Can you work these out from the model? Positions are in its coordinate system, mm. A direction names the side the tool comes from. Give positions to 0.01 mm unless a question says otherwise; leave off trailing zeros. Order: outer loops, then holes, each group sorted by start corner. A loop starts at its lowest first (then second) coordinate and runs counter-clockwise, first axis right, second up.
Item 1: I want a section at A-A, the plane y = 21.5. Write out the boundary of the cut face in (x, z), then the cut area to 3 significant figures.
Item 2: I want a section at B-B, the plane z = 3.75. Write out the boundary of the cut face in (x, y).
Item 3: If we mould it in two halves opening along Y, with no side actions, what happens to faces 1 (the flat face through (33, 0, 5.08)), 2 (the cylindrical face through (53.944, 47.249, 3.792)), 3 (the cylindrical face through (18.98, -15.5, 6.86)), 4 (the flat face through (48, 31, 2.54))? For each: +Y half, -Y half, draft (parallel to the pull), parting line (faces both ways), or undercut.
Item 4: I'm going to push flat-ended pins straight in: pin 1 Ø5.5 at (x, y) = (33, 2.5) entering from -Z; pin 2 Ø1.5 at (x, z) = (43.5, 1) entering from +Y; pin 3 Ø2 at (x, z) = (28.5, 3) entering from +Y; pin 4 Ø12 at (x, y) = (8, 10) entering from +Z. Where does each tip first touch, or does it pass through?
Item 5: Which directions (+Z, -Z, +X, -X, +Y, -Y) give clear straight access to the entire face, cutting with the end or side of a thin tool? Please do faces 5 (the cylindrical face through (9.436, 23.933, 0.764)), 6 (the cylindrical face through (23.98, 61.47, 3.79)), 7 (the flat face through (0, 24, 4)), 8 (the flat face through (49.32, 34.14, 6.33)).
Item 6: If I drill on line 1 along X through (y, z) = (23.5, 5.25); line 2 along Y through (x, z) = (43.5, 3); line 3 along Y through (x, z) = (17, 7.25), over which ranges is the centre line in solid material (lowest first)?
```python
from build123d import *

# Parameters (mm, degrees)
BOSS_EXTRUDE1_DEPTH     = 7.62
FILLET1_R               = 2.54
SKETCH4_W               = 10.16
SKETCH4_H               = 2.54
BOSS_EXTRUDE2_DEPTH     = 40.698655059
CUT_EXTRUDE1_DEPTH      = 92.035139481
CUT_EXTRUDE1_DEPTH_BACK = 92.035139481
SKETCH7_R               = 1.27
CUT_EXTRUDE2_DEPTH      = 92.212140759


with BuildPart() as part:
    # Sketch2 → Boss-Extrude1 (new body)
    with BuildSketch(Plane.XY):
        with BuildLine():
            Line((557.368573337, 914.592873905), (556.734884655, 913.276848696))
            Line((556.734884655, 913.276848696), (547.580835245, 917.684680294))
            Line((547.580835245, 917.684680294), (548.214523926, 919.000705503))
            ThreePointArc((548.214523926, 919.000705503), (548.458818056, 919.731374997), (548.513066645, 920.499889552))
            ThreePointArc((548.513066645, 920.499889552), (547.585939227, 924.379743345), (545.358485968, 927.689015574))
            ThreePointArc((545.358485968, 927.689015574), (538.788952643, 934.173311823), (531.958551893, 940.382216038))
            ThreePointArc((531.958551893, 940.382216038), (526.80512603, 942.791823737), (521.15870091, 942.097640216))
            ThreePointArc((521.15870091, 942.097640216), (515.269866914, 937.194322522), (513.062812413, 929.85608018))
            Line((513.062812413, 929.85608018), (513.062812413, 881.310664403))
            ThreePointArc((513.062812413, 881.310664403), (514.84238247, 877.01697918), (519.13757646, 875.241053792))
            Line((519.13757646, 875.241053792), (524.686345009, 875.245763006))
            ThreePointArc((524.686345009, 875.245763006), (526.769666342, 875.847420281), (528.214212618, 877.464672677))
            Line((528.214212618, 877.464672677), (529.924061844, 881.015635083))
            Line((529.924061844, 881.015635083), (539.078111254, 876.607803485))
            Line((539.078111254, 876.607803485), (537.368262028, 873.056841079))
            ThreePointArc((537.368262028, 873.056841079), (532.178962974, 867.247123196), (524.69496775, 865.085766665))
            Line((524.69496775, 865.085766665), (519.146199201, 865.081057451))
            ThreePointArc((519.146199201, 865.081057451), (507.66122682, 869.82972633), (502.902812413, 881.310664403))
            Line((502.902812413, 881.310664403), (502.902812413, 929.85608018))
            ThreePointArc((502.902812413, 929.85608018), (506.79547726, 942.798813577), (517.181834766, 951.446978999))
            ThreePointArc((517.181834766, 951.446978999), (528.398937465, 952.826033478), (538.636655301, 948.039143286))
            ThreePointArc((538.636655301, 948.039143286), (545.776010677, 941.549396152), (552.642698999, 934.771800374))
            ThreePointArc((552.642698999, 934.771800374), (556.88965456, 928.462203511), (558.657354478, 921.064711969))
            ThreePointArc((558.657354478, 921.064711969), (558.423168364, 917.747106133), (557.368573337, 914.592873905))
        make_face()
    extrude(amount=BOSS_EXTRUDE1_DEPTH)


with BuildPart() as part_1:
    # Body-Move/Copy1: moved
    add(part.part.moved(Location((-502.902812413, -881.310664403, 0))))

    # Fillet1
    fillet1_edges = [part_1.edges().sort_by_distance(p)[0] for p in [
        (42.873198264, 60.238731749, 7.62),
        (53.986842147, 47.151539108, 7.62),
        (55.520355951, 36.43644173, 7.62),
        (54.148916583, 32.624196898, 7.62),
        (0, 24.272707889, 0),
        (4.758414407, -11.480938073, 0),
        (19.017771063, -16.227252345, 0),
        (29.276150561, -14.063541207, 0),
        (35.320374228, -6.478342121, 0),
        (26.166324818, -2.070510523, 0),
        (23.86685393, -5.463244122, 0),
        (19.009148321, -6.067256004, 0),
        (11.939570057, -4.293685223, 0),
        (10.16, 24.272707889, 0),
        (12.367054501, 55.883658119, 0),
        (44.994867173, 37.032028495, 7.62),
        (23.902313617, 61.481159334, 0),
        (35.88614023, 52.86264742, 0),
        (44.683126814, 43.069078942, 0),
        (45.556005643, 38.420710594, 0),
        (44.994867173, 37.032028495, 0),
        (54.148916583, 32.624196898, 0),
        (45.556005643, 38.420710594, 7.62),
        (55.520355951, 36.43644173, 0),
        (53.986842147, 47.151539108, 0),
        (42.873198264, 60.238731749, 0),
        (25.496125052, 71.515369074, 0),
        (3.892664847, 61.488149174, 0),
        (44.683126814, 43.069078942, 7.62),
        (35.88614023, 52.86264742, 7.62),
        (23.902313617, 61.481159334, 7.62),
        (3.892664847, 61.488149174, 7.62),
        (12.367054501, 55.883658119, 7.62),
        (10.16, 24.272707889, 7.62),
        (11.939570057, -4.293685223, 7.62),
        (19.009148321, -6.067256004, 7.62),
        (23.86685393, -5.463244122, 7.62),
        (26.166324818, -2.070510523, 7.62),
        (35.320374228, -6.478342121, 7.62),
        (29.276150561, -14.063541207, 7.62),
        (19.017771063, -16.227252345, 7.62),
        (25.496125052, 71.515369074, 7.62),
        (4.758414407, -11.480938073, 7.62),
        (0, 24.272707889, 7.62),
    ]]
    fillet(fillet1_edges, radius=FILLET1_R)

    # Sketch4 → Boss-Extrude2 (add)
    with BuildSketch(Plane(origin=(22.627352506, 46.991791376, 0), x_dir=(0.9009891151809732, -0.433841692700698, 0), z_dir=(-0.43384169270069806, -0.9009891151809734, 0))):
        with Locations((29.553847635, 3.81)):
            Rectangle(SKETCH4_W, SKETCH4_H)
    extrude(amount=BOSS_EXTRUDE2_DEPTH)

    # Sketch5 → Cut-Extrude1 (cut, two sides: drawn at the far end of the back side and taken through both)
    with BuildSketch(Plane.XY.offset(5.08).offset(-CUT_EXTRUDE1_DEPTH_BACK)):
        Polygon((41.372149134, 29.508478833), (50.526198544, 25.100647236), (39.48117254, 2.16267614), (30.327123129, 6.570507738), align=None)
    extrude(amount=CUT_EXTRUDE1_DEPTH + CUT_EXTRUDE1_DEPTH_BACK, mode=Mode.SUBTRACT)

    # Sketch7 → Cut-Extrude2 (cut, through all)
    with BuildSketch(Plane.XY):
        with Locations(Location((33.802189935, 2.078079586, 0), (0, 0, 180))):
            Circle(SKETCH7_R)
    extrude(amount=CUT_EXTRUDE2_DEPTH, mode=Mode.SUBTRACT)


solid = part_1.part
```
Results list:
1. outline: (0, 2.54) arc R2.54 ccw to (2.54, 0) - (7.62, 0) arc R2.54 ccw to (10.16, 2.54) - (10.16, 5.08) arc R2.54 ccw to (7.62, 7.62) - (2.54, 7.62) arc R2.54 ccw to (0, 5.08) - close
1. area: 71.9 mm2
2. outline: (0, 0) arc R16.23 ccw to (16.24, -16.23) - (21.79, -16.22) arc R14.08 ccw to (34.47, -8.25) - (39.48, 2.16) - (30.33, 6.57) - (25.31, -3.85) arc R3.92 cw to (21.78, -6.06) - (16.23, -6.07) arc R6.07 cw to (10.16, 0) - (10.16, 48.55) arc R13.3 cw to (18.26, 60.79) arc R10.3 cw to (29.06, 59.07) arc R224.62 cw to (42.46, 46.38) arc R11.21 cw to (45.61, 39.19) arc R3.06 cw to (45.31, 37.69) - (41.37, 29.51) - (50.53, 25.1) - (54.47, 33.28) arc R13.22 ccw to (55.75, 39.75) arc R21.37 ccw to (49.74, 53.46) arc R234.78 ccw to (35.73, 66.73) arc R20.46 ccw to (14.28, 70.14) arc R23.46 ccw to (0, 48.55) - close; hole circle Ø2.54 at (33.8, 2.08)
3. face 1: undercut
3. face 2: +Y half
3. face 3: -Y half
3. face 4: draft
4. pin 1: stops at z = 2.54
4. pin 2: stops at y = 59.88
4. pin 3: stops at y = 71.09
4. pin 4: stops at z = 7.62
5. face 5: -Z
5. face 6: +Z, -Z
5. face 7: +Z, -Z, -X, +Y, -Y
5. face 8: +Z, -Y
6. line 1: x = 0.01 to 10.15
6. line 2: y = 28.48 to 33.93, 45.14 to 59.64
6. line 3: y = -15.01 to -7.29, 61.55 to 69.81
